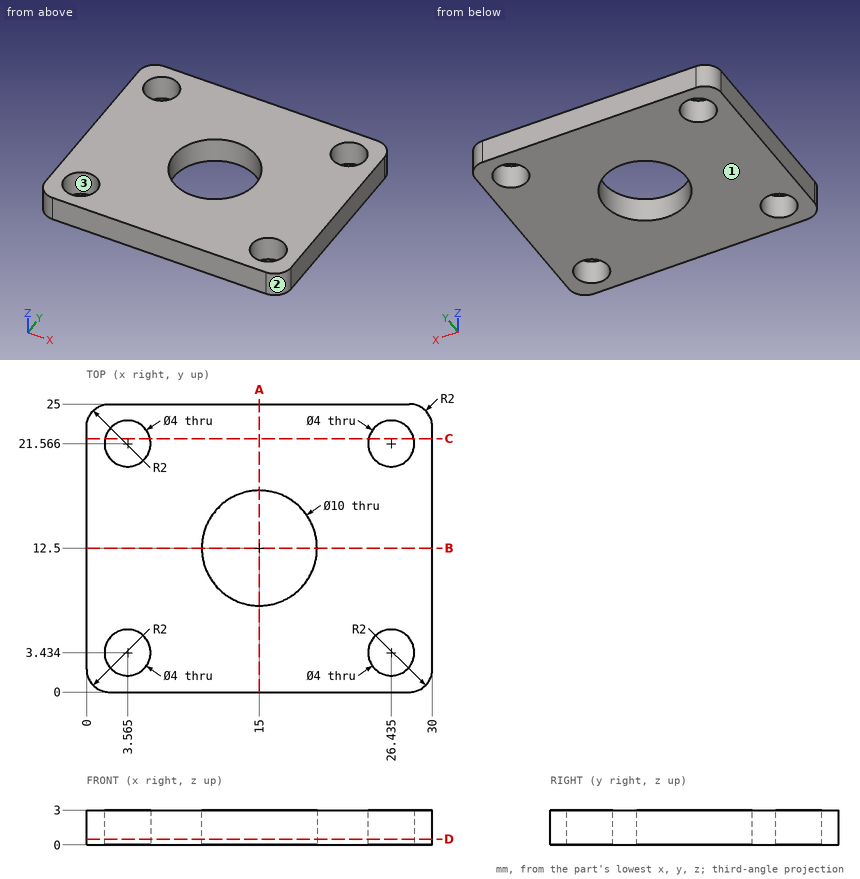
Geometry check sheet. Reference: drawing and pictorial views, mm from the part's lowest x, y, z. Give positions to 0.01 mm unless a question says otherwise; leave off trailing zeros. Order: outer loops, then holes, each group sorted by start corner. A loop starts at its lowest first (then second) coordinate and runs counter-clockwise, first axis right, second up. Notation, with made-up numbers: (59.25, -28.5) - (70.25, -28.5) arc R21 cw to (70.25, -24.5) - close; hole circle Ø11 at (9.5, 72). An arc over 180 degrees is marked (long way). Answer as CSV lines item,"result".
1. Section check B-B (y = 12.5). Record the boundary of the cut face in (x, z), then the cut area to 3 significant figures.
Result sheet:
outline,"(0, 0) - (10, 0) - (10, 3) - (0, 3) - close; (20, 0) - (30, 0) - (30, 3) - (20, 3) - close"
area,"60.0 mm²"
2. Mould release check, pull along Y, two halves, no side actions. Record for the marked faces 1, 2 and 3: released by +Y, released by -Y, zero draft, split by the parting line, or undercut.
Result sheet:
face 1,"zero draft"
face 2,"released by -Y"
face 3,"undercut"
3. Section check C-C (y = 22). Record the boundary of the cut face in (x, z).
Result sheet:
outline,"(0, 0) - (1.61, 0) - (1.61, 3) - (0, 3) - close; (5.52, 0) - (24.48, 0) - (24.48, 3) - (5.52, 3) - close; (28.39, 0) - (30, 0) - (30, 3) - (28.39, 3) - close"
4. Scan lines: probe 1 along X at (y, z) = (22, 2.65); probe 2 along X at (y, z) = (4.25, 0.5); probe 3 along Y at (x, z) = (26, 2.45). Record each from-to range of solid material in increasing order. Write a range as from..to.
Result sheet:
probe 1,"0..1.61, 5.52..24.48, 28.39..30"
probe 2,"0..1.74, 5.39..24.61, 28.26..30"
probe 3,"0..1.48, 5.39..19.61, 23.52..25"
5. Section check D-D (z = 0.5). Record the boundary of the cut face in (x, y) (1 decimal), then the cut area to 3 significant figures.
Result sheet:
outline,"(0, 2) arc R2 ccw to (2, 0) - (28, 0) arc R2 ccw to (30, 2) - (30, 23) arc R2 ccw to (28, 25) - (2, 25) arc R2 ccw to (0, 23) - close; hole circle Ø4 at (3.6, 3.4); hole circle Ø4 at (3.6, 21.6); hole circle Ø10 at (15, 12.5); hole circle Ø4 at (26.4, 3.4); hole circle Ø4 at (26.4, 21.6)"
area,"618 mm²"
6. Section check A-A (x = 15). Record the boundary of the cut face in (y, z), then the cut area to 3 significant figures.
Result sheet:
outline,"(0, 0) - (7.5, 0) - (7.5, 3) - (0, 3) - close; (17.5, 0) - (25, 0) - (25, 3) - (17.5, 3) - close"
area,"45.0 mm²"
